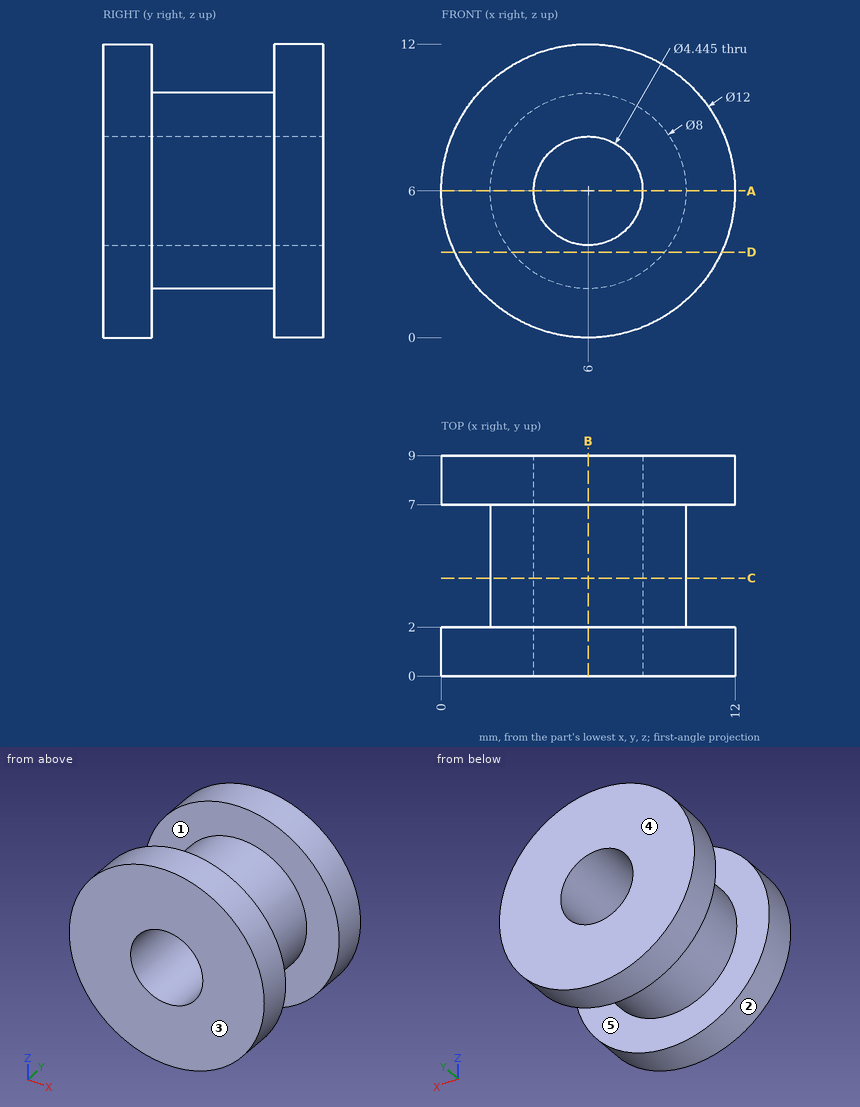
Here's the drawing with two shaded views (mm, measured from the low corner). I have some questions. A direction names the side the tool comes from. Round coordinates to 2 decimals unless told otherwise and drop trailing zeros. Loops run counter-clockwise (first coordinate to the right, second up) from the corner with the lowest first, then second, coordinate; pieces in that order, holes last. Notation, with made-up numbers: M 68.25,25 L 92.25,25 A18 ccw 92.25,30 Z; hole C 38.25,26 d2. An arc over 180 degrees is marked long. Answer as a JSON object with one key per item and string values. Group by question number.
Q1. Please list where these lines run through material, in increasing order: L1, parallel to Y at x = 2.25, z = 10.5; L2, parallel to Z at x = 6, y = 5.75.
Q2. On a 3-axis mill with a long thin cutter (end or side, diameter ignored), from which of +Z, -Z, +X, -X, +Y, -Y can I reach the whole of each face in a straight line? I mean the marked faces 1 and 2. Say none if no direction works.
Q3. Imagine slicing it at C-C, the plane y = 4. Please give me the cut outline in (x, z) (1 decimal).
Q4. We'd pull the mould along Y, two halves only. Please class the marked faces 3, 4 and 5: +Y half, -Y half, draft (parallel to the pull), parting line (faces both ways), or undercut.
Q5. Imagine slicing it at D-D, the plane z = 3.5. Please give me the cut outline in (x, y).
Q6. Imagine slicing it at B-B, the plane x = 6. Please give me the cut outline in (y, z), then the cut area to 3 significant figures.
Q7. Will these pins go through, and if not, where does the flat tip stop? pin 1 (6 mm diameter, centred on x = 5, z = 4, fed in from -Y); pin 2 (4 mm diameter, centred on x = 1.5, y = 7.5, fed in from +Z); pin 3 (1.5 mm diameter, centred on y = 3.5, z = 6, fed in from +X); pin 4 (2.5 mm diameter, centred on x = 6, z = 6, fed in from -Y).
Q8. Imagine slicing it at A-A, the plane z = 6. Please give me the cut outline in (x, y), then the cut area to 3 significant figures.
Findings:
{
 "1": {"L1": "y = 0 to 2, 7 to 9", "L2": "z = 2 to 3.78, 8.22 to 10"},
 "2": {"face 1": "none", "face 2": "+Y, -Y"},
 "3": {"outline": "C 6,6 d8; hole C 6,6 d4.4"},
 "4": {"face 3": "-Y half", "face 4": "+Y half", "face 5": "undercut"},
 "5": {"outline": "M 0.55,0 L 11.45,0 L 11.45,2 L 9.12,2 L 9.12,7 L 11.45,7 L 11.45,9 L 0.55,9 L 0.55,7 L 2.88,7 L 2.88,2 L 0.55,2 Z"},
 "6": {"outline": "M 0,0 L 2,0 L 2,2 L 7,2 L 7,0 L 9,0 L 9,3.78 L 0,3.78 Z; M 0,8.22 L 9,8.22 L 9,12 L 7,12 L 7,10 L 2,10 L 2,12 L 0,12 Z", "area": "48.0 mm2"},
 "7": {"pin 1": "stops at y = 0", "pin 2": "stops at z = 11.45", "pin 3": "stops at x = 10", "pin 4": "passes through"},
 "8": {"outline": "M 0,0 L 3.78,0 L 3.78,9 L 0,9 L 0,7 L 2,7 L 2,2 L 0,2 Z; M 8.22,0 L 12,0 L 12,2 L 10,2 L 10,7 L 12,7 L 12,9 L 8.22,9 Z", "area": "48.0 mm2"}
}
